Here's how the part is built. I have some questions about the finished solid (model axes, mm). A direction names the side the tool comes from. Round coordinates to 2 decimals unless told otherwise and drop trailing zeros. Loops run counter-clockwise (first coordinate to the right, second up) from the corner with the lowest first, then second, coordinate; pieces in that order, holes last. Notation, with made-up numbers: M 46,79.25 L 98,79.25 A10 ccw 98,93.25 Z; hole C 68.5,33.5 d7. An arc over 180 degrees is marked long. Answer as CSV lines item,"result".
Autodesk Inventor part; units mm, degrees
ref_plane "YZ Plane" through (0, 0, 0) normal (1, 0, 0) x (0, 1, 0)
ref_plane "XZ Plane" through (0, 0, 0) normal (0, 1, 0) x (-1, 0, 0)
ref_plane "XY Plane" through (0, 0, 0) normal (0, 0, 1) x (1, 0, 0)
sketch "Sketch1" plane through (0, 0, 0) normal (0, 0, 1) x (1, 0, 0)
  line L0 (0, 0) -> (25.4, 0)
  line L1 (25.4, 0) -> (25.4, 1.5875)
  line L2 (25.4, 1.5875) -> (1.5875, 1.5875)
  line L3 (0, 0) -> (0, 25.4)
  line L4 (0, 25.4) -> (1.5875, 25.4)
  line L5 (1.5875, 1.5875) -> (1.5875, 25.4)
  dimension "d0" = 25.4
  dimension "d1" = 1.5875
  dimension "d2" = 25.4
  dimension "d3" = 1.5875
extrude "Extrusion1" add sketch "Sketch1" along normal blind 1498.6
sketch "Sketch2" plane through (0, 0, 1498.6) normal (0, 0, 1) x (1, 0, 0)
  line L0 (0, 0) -> (25.4, 0)
  line L1 (25.4, 0) -> (25.4, 1.5875)
  line L2 (25.4, 1.5875) -> (1.5875, 1.5875)
  line L3 (1.5875, 1.5875) -> (1.5875, 25.4)
  line L4 (1.5875, 25.4) -> (0, 25.4)
  line L5 (0, 25.4) -> (0, 0)
extrude "Extrusion2" cut sketch "Sketch2" against normal blind 812.8 keep common part
properties part number "32-LBracketVersaFrame-1111-2018"
1. For P1, Ø7, axis at y = 9.5, z = 1145.5, coming from the +X side; P2, Ø12, axis at x = 8, z = 934, coming from the +Y side, each with a flat end and sliding along its axis, tell me the tip position at first contact or that it passes through.
Evaluation:
P1,"stops at x = 1.59"
P2,"stops at y = 1.59"
2. I want a section at C-C, the plane z = 908. Please give me the cut outline in (x, y), and give its area (3 significant figures).
Evaluation:
outline,"M 0,0 L 25.4,0 L 25.4,1.59 L 1.59,1.59 L 1.59,25.4 L 0,25.4 Z"
area,"78.1 mm²"
3. Which directions (+Z, -Z, +X, -X, +Y, -Y) give clear straight access to the entire face, cutting with the end or side of a thin tool? Please do faces 1 (the flat face through (1.588, 13, 1087)), 2 (the flat face through (1, 7, 1498.6)).
Evaluation:
face 1,"+Z, -Z, +X, +Y"
face 2,"+Z, +X, -X, +Y, -Y"
4. I want a section at A-A, the plane x = 13.25. Please give me the cut outline in (y, z).
Evaluation:
outline,"M 0,685.8 L 1.59,685.8 L 1.59,1498.6 L 0,1498.6 Z"
5. If I drill on line 1 (X direction, y = 5.75, z = 1380), over which ranges is the centre line in solid material (lowest first)? Write a range as [from, to].
Evaluation:
line 1,"x = [0, 1.59]"
